Autodesk Inventor part; units mm, degrees
ref_plane "YZ Plane" through (0, 0, 0) normal (1, 0, 0) x (0, 1, 0)
ref_plane "XZ Plane" through (0, 0, 0) normal (0, 1, 0) x (-1, 0, 0)
ref_plane "XY Plane" through (0, 0, 0) normal (0, 0, 1) x (1, 0, 0)
sketch "Sketch1" plane through (0, 0, 0) normal (1, 0, 0) x (0, 1, 0)
  line L0 (25346.4946, 38060.2067) -> (25328.8946, 38060.2067)
  line L1 (0, -1) -> (0, -18.6)
  line L2 (-15.25, -26.1) -> (-28.5, -26.1)
  line L3 (-15.25, 7.5) -> (-28.5, 7.5)
  line L4 (-15.25, 7.5) -> (0, -1)
  line L5 (0, -18.6) -> (-15.25, -26.1)
  line L6 (-28.5, 12.5) -> (-13.9507, 12.5)
  line L7 (-13.9507, 12.5) -> (5, 1.9373)
  line L8 (5, 1.9373) -> (5, -21.7129)
  line L9 (5, -21.7129) -> (-14.087, -31.1)
  line L10 (-14.087, -31.1) -> (-28.5, -31.1)
  line L11 (-28.5, 12.5) -> (-28.5, 7.5)
  line L12 (-28.5, -26.1) -> (-28.5, -31.1)
  dimension "d2" = 17.6
  dimension "d8" = 5
  dimension "d12" = 38.6
extrude "Extrusion1" add sketch "Sketch1" along normal blind 60
properties part number "BatteryHolder"
Verification items for the finished model (mm, model axes). A direction names the side the tool comes from. Round coordinates to 2 decimals unless told otherwise and drop trailing zeros. Write each loop counter-clockwise with the first axis right and the second up, starting at its lowest first coordinate (ties: lowest second). Pieces come first, ordered by that corner, then holes. Notation, with made-up numbers: (-24, -38.75) -> (-3, -38.75) arc R15 cw to (-3, -24.75) -> close; hole circle Ø9 at (84.5, -38.75). An arc over 180 degrees is marked (long way). Write each question's results on one line, items separated by ' | '.
Q1. Sectioned sample at D-D, the plane z = -2.5. Record the boundary of the cut face in (x, y).
Derived:
outline: (0, 0) -> (60, 0) -> (60, 5) -> (0, 5) -> close
Q2. Sectioned sample at A-A, the plane y = -16. Record the boundary of the cut face in (x, z).
Derived:
outline: (0, -31.1) -> (60, -31.1) -> (60, -26.1) -> (0, -26.1) -> close; (0, 7.5) -> (60, 7.5) -> (60, 12.5) -> (0, 12.5) -> close
Q3. Access from +Z, -Z, +X, -X, +Y, -Y to the whole of each face (thin tool, end or side, straight path). Record for faces 1 (the face through (29.58, -7.52, -22.3)), 2 (the face through (60, 1, -9)).
Derived:
face 1: +X, -X, -Y | face 2: +Z, -Z, +X, +Y, -Y
Q4. Go/stop test with flat-tipped pins: pin 1 Ø19.5 at (x, z) = (42, -9) entering from -Y; pin 2 Ø5 at (x, y) = (31.5, -6) entering from +Z; pin 3 Ø6 at (x, y) = (14.5, -9) entering from +Z. Record where each tip stops, or that it passes through.
Derived:
pin 1: stops at y = -3.14 | pin 2: stops at z = 9.46 | pin 3: stops at z = 11.41
Q5. Thickness scan on probe 1 along Z at (x, y) = (52, -20); probe 2 along Y at (x, z) = (11.5, -9); probe 3 along Z at (x, y) = (47.5, -3). Record the ranges inside material, lowest first.
Derived:
probe 1: z = -31.1 to -26.1, 7.5 to 12.5 | probe 2: y = 0 to 5 | probe 3: z = -25.65 to -20.08, 0.67 to 6.4
Q6. Sectioned sample at C-C, the plane y = -12. Record the boundary of the cut face in (x, z).
Derived:
outline: (0, -30.07) -> (60, -30.07) -> (60, -24.5) -> (0, -24.5) -> close; (0, 5.69) -> (60, 5.69) -> (60, 11.41) -> (0, 11.41) -> close
Q7. Sectioned sample at B-B, the plane x = 10. Record the boundary of the cut face in (y, z), and give its area (3 significant figures).
Derived:
outline: (-28.5, -31.1) -> (-14.09, -31.1) -> (5, -21.71) -> (5, 1.94) -> (-13.95, 12.5) -> (-28.5, 12.5) -> (-28.5, 7.5) -> (-15.25, 7.5) -> (0, -1) -> (0, -18.6) -> (-15.25, -26.1) -> (-28.5, -26.1) -> close | area: 435 mm²
